Verification items for this drawing (mm, ordinates from the low corner). A direction names the side the tool comes from. Give positions to 0.01 mm unless a question says otherwise; leave off trailing zeros. Order: outer loops, then holes, each group sorted by start corner. A loop starts at its lowest first (then second) coordinate and runs counter-clockwise, first axis right, second up. Notation, with made-up numbers: (-28.5, 37.5) -> (4.5, 37.5) arc R20 cw to (4.5, 64.5) -> close; hole circle Ø6 at (-12, 59). An arc over 180 degrees is marked (long way). One line per question, with ' | ' between items.
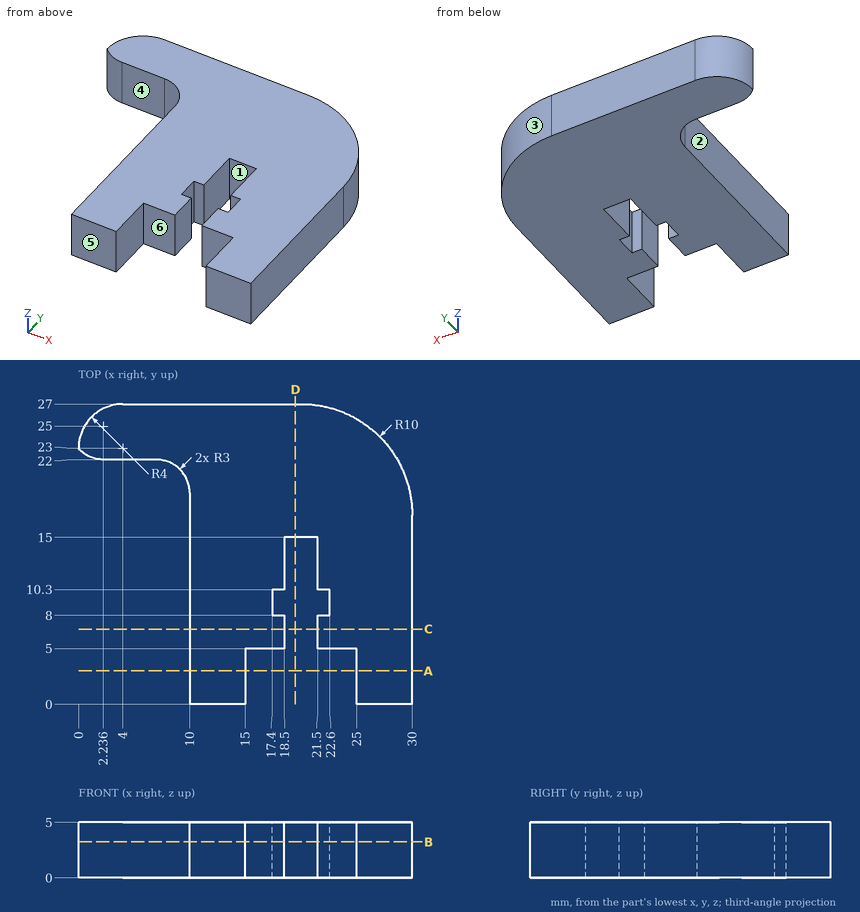
Q1. Section check B-B (z = 3.25). Enter the section's corners in (x, y), and give its area (3 significant figures).
Result sheet:
outline: (0, 23) arc R3 ccw to (2.24, 22) -> (7, 22) arc R3 cw to (10, 19) -> (10, 0) -> (15, 0) -> (15, 5) -> (18.5, 5) -> (18.5, 8) -> (17.4, 8) -> (17.4, 10.3) -> (18.5, 10.3) -> (18.5, 15) -> (21.5, 15) -> (21.5, 10.3) -> (22.6, 10.3) -> (22.6, 8) -> (21.5, 8) -> (21.5, 5) -> (25, 5) -> (25, 0) -> (30, 0) -> (30, 17) arc R10 ccw to (20, 27) -> (4, 27) arc R4 ccw to start | area: 481 mm2
Q2. Section check D-D (x = 19.5). Enter the section's corners in (y, z), and give its area (3 significant figures).
Result sheet:
outline: (15, 0) -> (27, 0) -> (27, 5) -> (15, 5) -> close | area: 60.0 mm2
Q3. Section check A-A (y = 3). Enter the section's corners in (x, z), and give its area (3 significant figures).
Result sheet:
outline: (10, 0) -> (15, 0) -> (15, 5) -> (10, 5) -> close; (25, 0) -> (30, 0) -> (30, 5) -> (25, 5) -> close | area: 50.0 mm2
Q4. Mould release check, pull along X, two halves, no side actions. Record for the marked faces 1, 2, 3 and 4: pulls with the +X half, pulls with the -X half, needs draft (parallel to the pull), parting line crosses it, or undercut.
Result sheet:
face 1: undercut | face 2: pulls with the -X half | face 3: pulls with the +X half | face 4: needs draft
Q5. Section check C-C (y = 6.75). Enter the section's corners in (x, z).
Result sheet:
outline: (10, 0) -> (18.5, 0) -> (18.5, 5) -> (10, 5) -> close; (21.5, 0) -> (30, 0) -> (30, 5) -> (21.5, 5) -> close
Q6. Depth check by flat-ended pin: pin 1 Ø1.2 at (y, z) = (8.5, 3.5) entering from -X; pin 2 Ø0.9 at (x, z) = (22, 2) entering from +Y; pin 3 Ø2.5 at (x, z) = (20.5, 1.5) entering from -Y. Enter the tip coordinate at first touch or a pass-through.
Result sheet:
pin 1: stops at x = 10 | pin 2: stops at y = 26.88 | pin 3: stops at y = 5
Q7. Access from +Z, -Z, +X, -X, +Y, -Y to the whole of each face (thin tool, end or side, straight path). Record for the marked faces 5 and 6.
Result sheet:
face 5: +Z, -Z, +X, -X, -Y | face 6: +Z, -Z, -Y
Q8. Thickness scan on line 1 (X direction, y = 9.75, z = 1.55); line 2 (X direction, y = 13.75, z = 3.6); line 3 (Y direction, x = 17.5, z = 4.05). Record the ranges inside material, lowest first.
Result sheet:
line 1: x = 10 to 17.4, 22.6 to 30 | line 2: x = 10 to 18.5, 21.5 to 30 | line 3: y = 5 to 8, 10.3 to 27
